Part print with two shaded views. Sizes in mm from the minimum x, y, z corner. Round coordinates to 2 decimals unless told otherwise and drop trailing zeros. Write each loop counter-clockwise with the first axis right and the second up, starting at its lowest first coordinate (ties: lowest second). Pieces come first, ordered by that corner, then holes. Notation, with made-up numbers: (-9.75, 75.25) -> (3.25, 75.25) arc R15 ccw to (3.25, 82.25) -> close; hole circle Ø7 at (88.25, 50.25). An arc over 180 degrees is marked (long way). Answer in a Markdown table with one row per item. Add a question column.
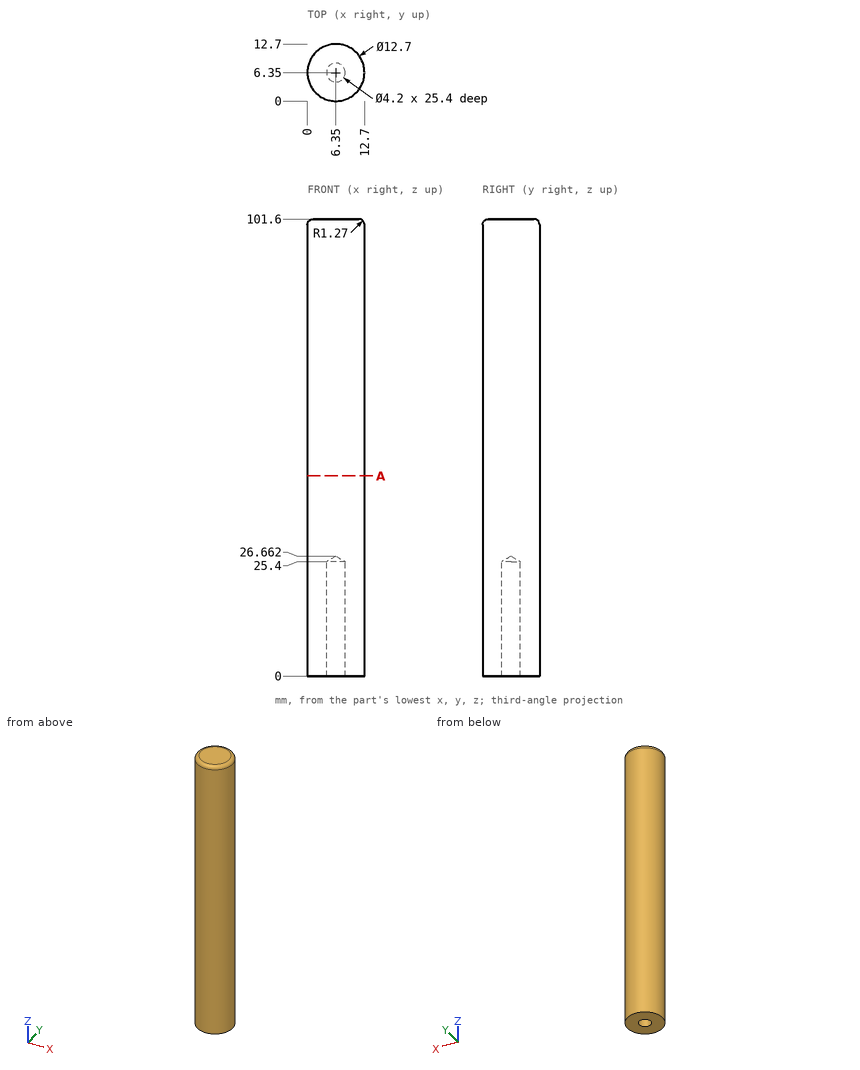
Item 1: Drill centre lines: probe 1 along Y at (x, z) = (6.35, 16); probe 2 along X at (y, z) = (6.75, 56); probe 3 along X at (y, z) = (4.75, 95) (1 decimal). Where is each one in solid material? Low to high.
Item 2: Pin check, flat tips, straight feed: pin 1 (1 mm diameter, centred on y = 4, z = 39, fed in from +X); pin 2 (1 mm diameter, centred on y = 4.5, z = 32, fed in from +X) (1 decimal); pin 3 (3 mm diameter, centred on x = 8.5, z = 32, fed in from -Y). Stop position of each tip, or through.
Item 3: Saw through at A-A on z = 44.5. Give the cut face in (x, y).
Recorded:
| question | item | result |
|---|---|---|
| 1 | probe 1 | 0 to 4.25, 8.45 to 12.7 |
| 1 | probe 2 | 0.01 to 12.69 |
| 1 | probe 3 | 0.2 to 12.5 |
| 2 | pin 1 | x = 12.42 |
| 2 | pin 2 | x = 12.6 |
| 2 | pin 3 | y = 0.03 |
| 3 | outline | circle Ø12.7 at (6.35, 6.35) |
